Can you work these out from the drawing? Everything is in mm from the part's minimum corner. A direction names the side the tool comes from. Round coordinates to 2 decimals unless told otherwise and drop trailing zeros. Loops run counter-clockwise (first coordinate to the right, second up) from the corner with the lowest first, then second, coordinate; pieces in that order, holes last. Notation, with made-up numbers: (37, 58.5) - (54, 58.5) arc R6 ccw to (54, 69.5) - close; hole circle Ø8 at (81.25, -3.75). An arc over 180 degrees is marked (long way). Answer as a JSON object with one key per item and string values. Group by question number.
1) I want a section at C-C, the plane x = 10. Please give me the cut outline in (y, z).
2) I want a section at A-A, the plane y = 4.75. Please give me the cut outline in (x, z), then the cut area to 3 significant figures.
3) Which directions (+Z, -Z, +X, -X, +Y, -Y) give clear straight access to the entire face, cutting with the end or side of a thin tool? Please do the marked faces 1 and 2.
4) If I drill on line 1 along X through (y, z) = (6, 4.5); line 2 along Z through (x, y) = (15.4, 1.55); line 3 along X through (y, z) = (4, 5.5), over which ranges is the centre line in solid material (lowest first)? Write a range as [from, to].
5) Will this pin go through, and if not, where does the flat tip stop? P1, Ø2.5, axis at x = 4, z = 4, coming from the +Y side.
6) If we mould it in two halves opening along X, with no side actions, what happens to the marked faces 3, 4 and 5? For each: pulls with the +X half, pulls with the -X half, needs draft (parallel to the pull), parting line crosses it, or undercut.
7) I want a section at D-D, the plane y = 1.5. Please give me the cut outline in (x, z), then the cut area to 3 significant figures.
8) I want a section at B-B, the plane z = 5. Please give me the cut outline in (x, y).
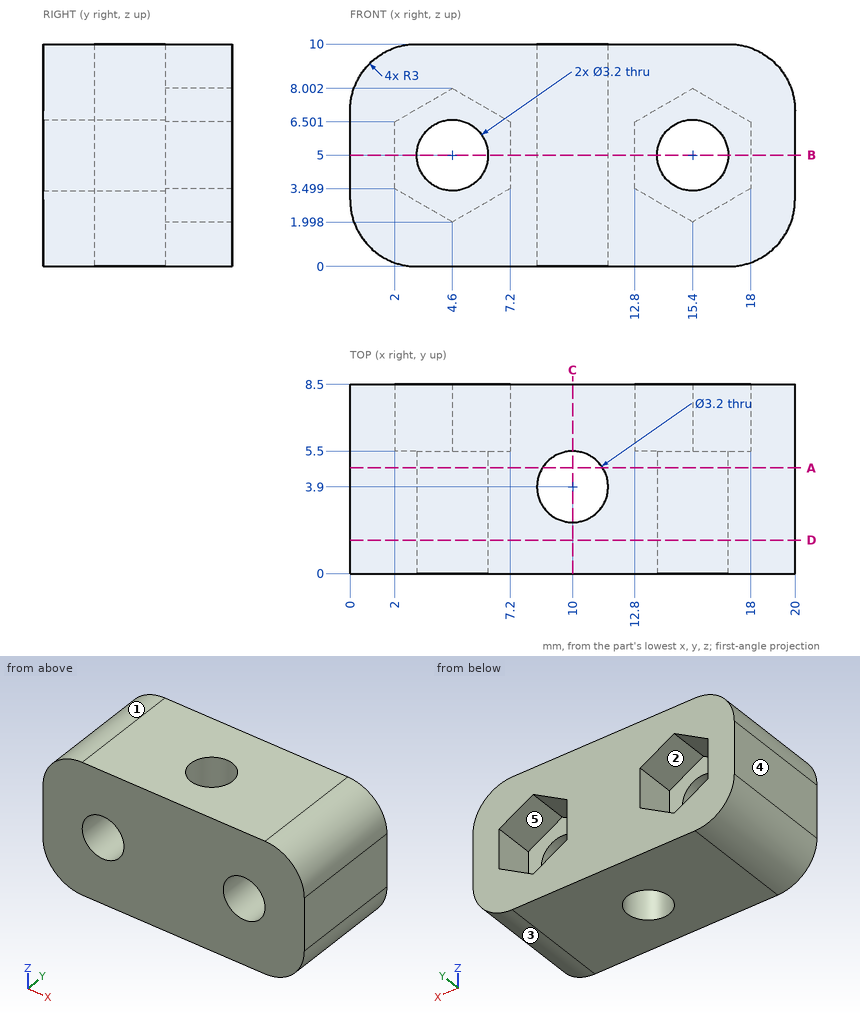
Outcome:
{
 "1": {"outline": "(0, 0) - (2.3, 0) - (2.3, 10) - (0, 10) - close; (5.5, 0) - (8.5, 0) - (8.5, 10) - (5.5, 10) - close"},
 "2": {"outline": "(0, 3) arc R3 ccw to (3, 0) - (8.64, 0) - (8.64, 10) - (3, 10) arc R3 ccw to (0, 7) - close; (11.36, 0) - (17, 0) arc R3 ccw to (20, 3) - (20, 7) arc R3 ccw to (17, 10) - (11.36, 10) - close; hole circle Ø3.2 at (4.6, 5); hole circle Ø3.2 at (15.4, 5)", "area": "149 mm^2"},
 "3": {"face 1": "+Z, -X, +Y, -Y", "face 2": "+Y"},
 "4": {"line 1": "[0, 2], [7.2, 12.8], [18, 20]", "line 2": "[0, 3.4], [6.6, 10]", "line 3": "[0, 3.08], [6.12, 8.4], [11.6, 13.88], [16.92, 20]"},
 "5": {"P1": "y = 5.5"},
 "6": {"face 3": "pulls with the +X half", "face 4": "pulls with the -X half", "face 5": "undercut"},
 "7": {"outline": "(0, 3) arc R3 ccw to (3, 0) - (17, 0) arc R3 ccw to (20, 3) - (20, 7) arc R3 ccw to (17, 10) - (3, 10) arc R3 ccw to (0, 7) - close; hole circle Ø3.2 at (4.6, 5); hole circle Ø3.2 at (15.4, 5)", "area": "176 mm^2"},
 "8": {"outline": "(0, 0) - (3, 0) - (3, 5.5) - (2, 5.5) - (2, 8.5) - (0, 8.5) - close; (6.2, 0) - (13.8, 0) - (13.8, 5.5) - (12.8, 5.5) - (12.8, 8.5) - (7.2, 8.5) - (7.2, 5.5) - (6.2, 5.5) - close; (17, 0) - (20, 0) - (20, 8.5) - (18, 8.5) - (18, 5.5) - (17, 5.5) - close; hole circle Ø3.2 at (10, 3.9)"}
}
